Part print with two shaded views. Sizes in mm from the minimum x, y, z corner. A direction names the side the tool comes from. Round coordinates to 2 decimals unless told otherwise and drop trailing zeros. Order: outer loops, then holes, each group sorted by start corner. A loop starts at its lowest first (then second) coordinate and runs counter-clockwise, first axis right, second up. Notation, with made-up numbers: M -3.5,45.5 L 53.5,45.5 A35 ccw 53.5,82.5 Z; hole C 1.25,18.5 d5. An arc over 180 degrees is marked long. Return JSON: item names as keys, results as strings. Group by question number.
Item 1: Slice it at D-D on y = 8.25. Write the cut outline in (x, z).
Item 2: Pin check, flat tips, straight feed: pin 1 Ø12 at (x, z) = (24.5, 17.5) entering from +Y; pin 2 Ø5 at (x, z) = (3, 19.5) entering from +Y; pin 3 Ø2 at (y, z) = (6, 34.5) entering from +X; pin 4 Ø4 at (x, y) = (20, 12) entering from -Z. Stop position of each tip, or through.
Item 3: Pull direction X, two halves, no side cores. Call the marked faces 3 and 4: pulls with the +X half, pulls with the -X half, needs draft (parallel to the pull), parting line crosses it, or undercut.
Item 4: Which spindle directions (+Z, -Z, +X, -X, +Y, -Y) get a long thin tool onto all of the face, cutting with end or side? Do the marked faces 1 and 2. Say none if no direction does.
Item 5: Slice it at C-C on z = 20.5. Write the cut outline in (x, y).
Item 6: Slice it at A-A on x = 20. Write the cut outline in (y, z), then the cut area to 4 significant figures.
Item 7: Probe line 1 along Y through (x, z) = (20, 0.65); line 2 along Y through (x, z) = (8.5, 13); line 3 along Z through (x, y) = (33.5, 11.5). List the from-to ranges inside material, lowest first.
Item 8: Slice it at B-B on y = 12. Write the cut outline in (x, z), then the cut area to 3 significant figures.
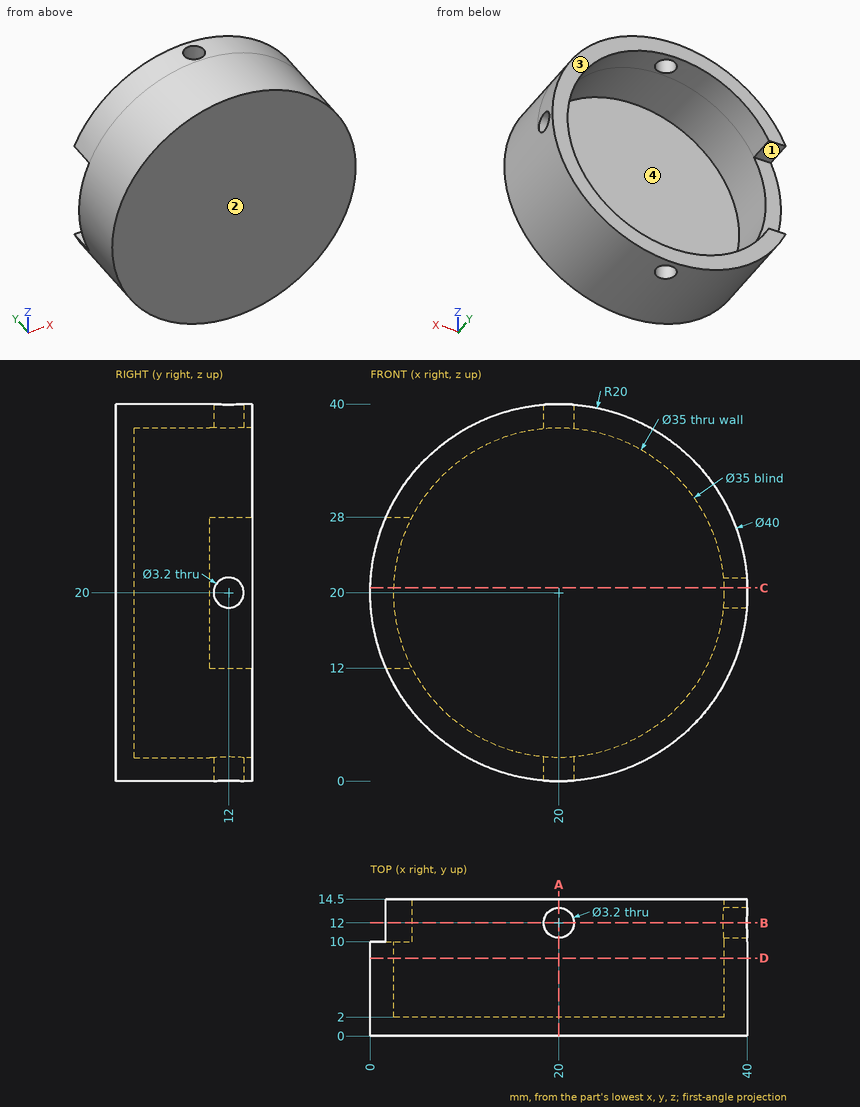
Output values:
{
 "1": {"outline": "C 20,20 d40; hole C 20,20 d35"},
 "2": {"pin 1": "y = 2", "pin 2": "y = 10", "pin 3": "x = 34.76", "pin 4": "z = 0"},
 "3": {"face 3": "needs draft", "face 4": "undercut"},
 "4": {"face 1": "-X, +Y", "face 2": "+Z, -Z, +X, -X, -Y"},
 "5": {"outline": "M 0.01,0 L 39.99,0 L 39.99,10.48 L 37.49,10.48 L 37.49,2 L 2.51,2 L 2.51,10 L 0.01,10 Z; M 37.49,13.52 L 39.99,13.52 L 39.99,14.5 L 37.49,14.5 Z"},
 "6": {"outline": "M 0,0 L 10.4,0 L 10.4,2.5 L 2,2.5 L 2,37.5 L 10.4,37.5 L 10.4,40 L 0,40 Z; M 13.6,0 L 14.5,0 L 14.5,2.5 L 13.6,2.5 Z; M 13.6,37.5 L 14.5,37.5 L 14.5,40 L 13.6,40 Z", "area": "126.5 mm²"},
 "7": {"line 1": "0 to 10.4, 13.6 to 14.5", "line 2": "0 to 2", "line 3": "5.24 to 8.86, 31.14 to 34.76"},
 "8": {"outline": "M 1.67,12 A20 ccw 18.4,0.06 L 18.4,2.57 A17.5 cw 4.44,12 Z; M 1.67,28 L 4.44,28 A17.5 cw 18.4,37.43 L 18.4,39.94 A20 ccw Z; M 21.6,0.06 A20 ccw 39.94,18.4 L 37.43,18.4 A17.5 cw 21.6,2.57 Z; M 21.6,37.43 A17.5 cw 37.43,21.6 L 39.94,21.6 A20 ccw 21.6,39.94 Z", "area": "229 mm²"}
}
